from build123d import *

# Parameters (mm, degrees)
SKETCH1_W           = 8.000974829
SKETCH1_H           = 46.5
BOSS_EXTRUDE1_DEPTH = 73
SKETCH2_R           = 11.15
CUT_EXTRUDE1_DEPTH  = 70
CUT_EXTRUDE3_DEPTH  = 62
SKETCH5_R           = 1.6
CUT_EXTRUDE4_DEPTH  = 62
FILLET2_START       = 8
FILLET2_DEPTH       = 60


with BuildPart() as part:
    # Sketch1 → Boss-Extrude1 (new body)
    with BuildSketch(Plane.XY):
        with Locations((34.458782271, 0)):
            Rectangle(SKETCH1_W, SKETCH1_H)
    extrude(amount=BOSS_EXTRUDE1_DEPTH)

    # Sketch2 → Cut-Extrude1 (cut)
    with BuildSketch(Plane(origin=(38.459269685, 0, 0), x_dir=(0, 0, -1), z_dir=(1, 0, 0))):
        with Locations((-58.8, 0)):
            Circle(SKETCH2_R)
        with BuildLine():
            Line((-73, -23.25), (-4.675968949, -23.25))
            ThreePointArc((-4.675968949, -23.25), (-5.84025075, -23.181991134), (-6.988696254, -22.978889578))
            Line((-6.988696254, -22.978889578), (-52.052198848, -12.266506414))
            ThreePointArc((-52.052198848, -12.266506414), (-63.616991815, -13.14521167), (-71.875840062, -5.002240165))
            Line((-71.875840062, -5.002240165), (-73, -8))
            Line((-73, -8), (-73, -23.25))
        make_face()
        with BuildLine():
            Line((-73, 23.25), (-73, 8))
            Line((-73, 8), (-71.875840062, 5.002240165))
            ThreePointArc((-71.875840062, 5.002240165), (-63.616991815, 13.14521167), (-52.052198848, 12.266506414))
            Line((-52.052198848, 12.266506414), (-6.988696254, 22.978889578))
            ThreePointArc((-6.988696254, 22.978889578), (-5.84025075, 23.181991134), (-4.675968949, 23.25))
            Line((-4.675968949, 23.25), (-73, 23.25))
        make_face()
        with BuildLine():
            Line((-73, 8), (-73, -8))
            Line((-73, -8), (-71.875840062, -5.002240165))
            ThreePointArc((-71.875840062, -5.002240165), (-72.8, 0), (-71.875840062, 5.002240165))
            Line((-71.875840062, 5.002240165), (-73, 8))
        make_face()
        with BuildLine():
            add(Edge.make_bspline(
                [(-5.680368735, -3.40627966), (-11.386784663, -11.746039667), (-21.714178832, -13.021085274)],
                knots=[0, 0, 0, 1, 1, 1], degree=2))
            add(Edge.make_bspline(
                [(-5.680368735, -3.40627966), (-15.724909711, -4.511710031), (-21.714178832, -13.021085274)],
                knots=[0, 0, 0, 1, 1, 1], degree=2))
        make_face()
        with BuildLine():
            add(Edge.make_bspline(
                [(-36.048150351, 0), (-23.713645553, 8.388071288), (-11.218940507, 0)],
                knots=[0, 0, 0, 1, 1, 1], degree=2))
            add(Edge.make_bspline(
                [(-36.048150351, 0), (-23.713645553, -8.388071288), (-11.218940507, 0)],
                knots=[0, 0, 0, 1, 1, 1], degree=2))
        make_face()
        with BuildLine():
            add(Edge.make_bspline(
                [(-5.680368735, 3.40627966), (-15.724909711, 4.511710031), (-21.714178832, 13.021085274)],
                knots=[0, 0, 0, 1, 1, 1], degree=2))
            add(Edge.make_bspline(
                [(-5.680368735, 3.40627966), (-11.386784663, 11.746039667), (-21.714178832, 13.021085274)],
                knots=[0, 0, 0, 1, 1, 1], degree=2))
        make_face()
    extrude(amount=-CUT_EXTRUDE1_DEPTH, mode=Mode.SUBTRACT)

    # Sketch4 → Cut-Extrude3 (cut)
    with BuildSketch(Plane.XY.offset(70)):
        with BuildLine():
            ThreePointArc((37.397007822, -19.25), (36.536421482, -17.172360788), (34.458782271, -16.311774449))
            Line((34.458782271, -16.311774449), (30.458294856, -16.311774449))
            Line((30.458294856, -16.311774449), (30.458294856, -22.188225551))
            Line((30.458294856, -22.188225551), (30.458294856, -24.738187672))
            Line((30.458294856, -24.738187672), (37.397007822, -23.25))
            Line((37.397007822, -23.25), (37.397007822, -19.25))
        make_face()
        with BuildLine():
            Line((30.458294856, 24.500594278), (30.458294856, 22.188225551))
            Line((30.458294856, 22.188225551), (30.458294856, 16.311774449))
            Line((30.458294856, 16.311774449), (34.458782271, 16.311774449))
            ThreePointArc((34.458782271, 16.311774449), (36.536421482, 17.172360788), (37.397007822, 19.25))
            Line((37.397007822, 19.25), (37.397007822, 23.25))
            Line((37.397007822, 23.25), (30.458294856, 24.500594278))
        make_face()
    extrude(amount=-CUT_EXTRUDE3_DEPTH, mode=Mode.SUBTRACT)

    # Sketch5 → Cut-Extrude4 (cut)
    with BuildSketch(Plane.XY.offset(8)):
        with Locations((34.458782271, 19.25)):
            Circle(SKETCH5_R)
        with Locations((34.458782271, -19.25)):
            Circle(SKETCH5_R)
    extrude(amount=-CUT_EXTRUDE4_DEPTH, mode=Mode.SUBTRACT)

    # Fillet2: read off the stored shape, not the designer's step
    # Fillet2 outline → Fillet2 (cut)
    with BuildSketch(Plane.XY.offset(FILLET2_START)):
        with BuildLine():
            ThreePointArc((34.828738175, -16.33515832), (31.706776269, -14.680417252), (30.458294856, -11.374950824))
            Line((30.458294856, -11.374950824), (30.458294856, -16.311774449))
            Line((30.458294856, -16.311774449), (34.458782271, -16.311774449))
            ThreePointArc((34.458782271, -16.311774449), (34.644129362, -16.317626244), (34.828738175, -16.33515832))
        make_face()
        with BuildLine():
            Line((30.458294856, 16.311774449), (30.458294856, 11.374950826))
            ThreePointArc((30.458294856, 11.374950826), (31.70677627, 14.680417253), (34.828738175, 16.33515832))
            ThreePointArc((34.828738175, 16.33515832), (34.644129362, 16.317626244), (34.458782271, 16.311774449))
            Line((34.458782271, 16.311774449), (30.458294856, 16.311774449))
        make_face()
    extrude(amount=FILLET2_DEPTH, mode=Mode.SUBTRACT)


solid = part.part
Can you work these out from the model? Positions are in its coordinate system, mm. A direction names the side the tool comes from. Give positions to 0.01 mm unless a question says otherwise; leave off trailing zeros. Loops run counter-clockwise (first coordinate to the right, second up) from the corner with the lowest first, then second, coordinate; pieces in that order, holes last. Notation, with made-up numbers: (59.5, 72.5) - (110.5, 72.5) arc R22 ccw to (110.5, 109.5) - close; hole circle Ø7 at (-36.75, 77.25). An arc over 180 degrees is marked (long way). Return JSON: item names as keys, results as strings.
1. We'd pull the mould along Y, two halves only. Please class faces 1 (the face through (34.51, 0.49, 69.94)), 2 (the face through (35.404, 15.167, 39.85)), 3 (the face through (35.404, -15.317, 39.219)): +Y half, -Y half, draft (parallel to the pull), parting line (faces both ways), or undercut.
Output values:
{"face 1": "undercut", "face 2": "+Y half", "face 3": "-Y half"}
2. I'm going to push flat-ended pins straight in: pin 1 Ø3 at (x, z) = (36, 65) entering from +Y; pin 2 Ø1 at (y, z) = (-21.5, 12) entering from -X. Where does each tip first touch, or does it pass through?
Output values:
{"pin 1": "stops at y = 13.19", "pin 2": "stops at x = 37.4"}
3. I want a section at A-A on z = 58.8. Please give me the cut outline in (x, y).
Output values:
{"outline": "(30.46, -11.37) arc R5 ccw to (31.2, -14) - (38.46, -14) - (38.46, -11.15) - (30.46, -11.15) - close; (30.46, 11.15) - (38.46, 11.15) - (38.46, 14) - (31.2, 14) arc R5 ccw to (30.46, 11.37) - close"}
4. For faces 4 (the face through (36.644, 17.285, 18.664)), 5 (the face through (33, -18, 8)), 6 (the face through (34.515, -23.184, 5.824)), which set-ups out of +Z, -Z, +X, -X, +Y, -Y let a thin tool reach every point of the face, with its end or its side?
Output values:
{"face 4": "+Z, -X, +Y", "face 5": "+Z, -X, -Y", "face 6": "+Z, +X, -X, -Y"}
5. I want a section at D-D on z = 44. Please give me the cut outline in (x, y), and give its area (3 significant figures).
Output values:
{"outline": "(30.46, -11.37) arc R5 ccw to (31.32, -14.18) - (38.46, -14.18) - (38.46, 14.18) - (31.32, 14.18) arc R5 ccw to (30.46, 11.37) - close", "area": "225 mm²"}
6. I want a section at B-B on x = 34. Give the number of separate pieces and of enclosed holes in the cut face, and give its area (3 significant figures).
Output values:
{"separate pieces": "3", "enclosed holes": "4", "area": "1,540 mm²"}
7. If I drill on line 1 (Z direction, x = 34.5, y = -2.5); line 2 (Z direction, x = 33, y = 9); line 3 (Y direction, x = 31, z = 9.5), over which ranges is the centre line in solid material (lowest first)?
Output values:
{"line 1": "z = 0 to 15.77, 31.55 to 47.93, 69.67 to 72.57", "line 2": "z = 0 to 11.06, 18.22 to 52.22, 65.38 to 69.52", "line 3": "y = -13.64 to -7.76, -4.13 to 4.13, 7.76 to 13.64"}
